The listing builds one solid part. Answer for the finished solid, in the listing's coordinates (mm). A direction names the side the tool comes from. Coordinates: 2 decimals unless noted, no trailing zeros. Write each loop counter-clockwise with the first axis right and the second up, starting at its lowest first coordinate (ties: lowest second). Pieces come first, ordered by that corner, then holes.
```python
from build123d import *

# Parameters (mm, degrees)
F1_DEPTH  = 5
F3_DEPTH  = 5.5
F5_DEPTH  = 5.5
F6_R      = 22.5
F7_DEPTH  = 10.5
F8_R      = 17.5
F9_DEPTH  = 25
F11_DEPTH = 25
F12_R     = 1.25
F13_DEPTH = 11
F14_R     = 2.25
F15_DEPTH = 2.5


with BuildPart() as f1:
    # F0 (on Top) → F1 (new body)
    with BuildSketch(Plane.XY):
        with BuildLine():
            Line((50.7170443075, -14.5414772037), (55.9852813742, -14.5414772037))
            Line((55.9852813742, -14.5414772037), (16.9705627485, 103))
            ThreePointArc((16.9705627485, 103), (8.4852813742, 109), (0, 103))
            Line((0, 103), (-39.0147186258, -14.5414772037))
            Line((-39.0147186258, -14.5414772037), (-33.746481559, -14.5414772037))
            Line((-33.746481559, -14.5414772037), (4.7271265323, 101.3697708508))
            ThreePointArc((4.7271265323, 101.3697708508), (8.4852813742, 104), (12.2434362162, 101.3697708508))
            Line((12.2434362162, 101.3697708508), (50.7170443075, -14.5414772037))
        make_face()
        with BuildLine():
            Line((16.9705627485, 103), (55.9852813742, -14.5414772037))
            Line((55.9852813742, -14.5414772037), (61.253518441, -14.5414772037))
            Line((61.253518441, -14.5414772037), (21.7024158273, 104.6159892602))
            ThreePointArc((21.7024158273, 104.6159892602), (8.4852813742, 114), (-4.7318530788, 104.6159892602))
            Line((-4.7318530788, 104.6159892602), (-44.2829556925, -14.5414772037))
            Line((-44.2829556925, -14.5414772037), (-39.0147186258, -14.5414772037))
            Line((-39.0147186258, -14.5414772037), (0, 103))
            ThreePointArc((0, 103), (8.4852813742, 109), (16.9705627485, 103))
        make_face()
        with BuildLine():
            Line((-33.746481559, -14.5414772037), (50.7170443075, -14.5414772037))
            Line((50.7170443075, -14.5414772037), (12.2434362162, 101.3697708508))
            ThreePointArc((12.2434362162, 101.3697708508), (8.4852813742, 104), (4.7271265323, 101.3697708508))
            Line((4.7271265323, 101.3697708508), (-33.746481559, -14.5414772037))
        make_face()
    extrude(amount=F1_DEPTH)

    # F2 (on face) → F3 (join)
    with BuildSketch(Plane.XY.offset(5)):
        with BuildLine():
            Line((-39.0147186258, -14.5414772037), (0, 103))
            ThreePointArc((0, 103), (8.4852813742, 109), (16.9705627485, 103))
            Line((16.9705627485, 103), (55.9852813742, -14.5414772037))
            Line((55.9852813742, -14.5414772037), (61.253518441, -14.5414772037))
            Line((61.253518441, -14.5414772037), (21.7024158273, 104.6159892602))
            ThreePointArc((21.7024158273, 104.6159892602), (8.4852813742, 114), (-4.7318530788, 104.6159892602))
            Line((-4.7318530788, 104.6159892602), (-44.2829556925, -14.5414772037))
            Line((-44.2829556925, -14.5414772037), (-39.0147186258, -14.5414772037))
        make_face()
    extrude(amount=F3_DEPTH)

    # F4 (on face) → F5 (join)
    with BuildSketch(Plane.XY.offset(5)):
        with BuildLine():
            ThreePointArc((11.29925422, 101.0399792418), (8.4852813742, 103), (5.6713085285, 101.0399792418))
            Line((5.6713085285, 101.0399792418), (-32.6928341457, -14.5414772037))
            Line((-32.6928341457, -14.5414772037), (-27.424597079, -14.5414772037))
            Line((-27.424597079, -14.5414772037), (8.4852813742, 93.6459020283))
            Line((8.4852813742, 93.6459020283), (44.3951598274, -14.5414772037))
            Line((44.3951598274, -14.5414772037), (49.6633968942, -14.5414772037))
            Line((49.6633968942, -14.5414772037), (11.29925422, 101.0399792418))
        make_face()
    extrude(amount=F5_DEPTH)

    # F6 (on face) → F7 (join)
    with BuildSketch(Plane.XY.offset(5)):
        with BuildLine():
            Line((36.3787330735, 9.6099885954), (27.3452487141, 36.8255916626))
            ThreePointArc((27.3452487141, 36.8255916626), (8.4852813742, 43.9585227963), (-10.3746859657, 36.8255916626))
            Line((-10.3746859657, 36.8255916626), (-19.4081703251, 9.6099885954))
            ThreePointArc((-19.4081703251, 9.6099885954), (8.4852813742, -13.0414772037), (36.3787330735, 9.6099885954))
        make_face()
        with Locations((8.4852813742, 15.4585227963)):
            Circle(F6_R, mode=Mode.SUBTRACT)
    extrude(amount=F7_DEPTH)

    # F8 (on face) → F9 (cut)
    with BuildSketch(Plane.XY.offset(5)):
        with Locations((8.4852813742, 15.4585227963)):
            Circle(F8_R)
    extrude(amount=-F9_DEPTH, mode=Mode.SUBTRACT)

    # F10 (on face) → F11 (cut)
    with BuildSketch(Plane.XY.offset(5)):
        with BuildLine():
            Line((8.4852813742, 77.7740365146), (-1.5945371695, 47.4060932537))
            ThreePointArc((-1.5945371695, 47.4060932537), (8.4852813742, 48.9585227963), (18.5650999179, 47.4060932537))
            Line((18.5650999179, 47.4060932537), (8.4852813742, 77.7740365146))
        make_face()
    extrude(amount=-F11_DEPTH, mode=Mode.SUBTRACT)

    # F12 (on face) → F13 (cut)
    with BuildSketch(Plane.XY.offset(10.5)):
        with Locations((8.4959140697, 97.6459020283)):
            Circle(F12_R)
        with Locations((-1.5147186258, 103.6459020283)):
            Circle(F12_R)
        with Locations((18.4852813742, 103.6459020283)):
            Circle(F12_R)
        with Locations((-10.2829556925, 45.4585227963)):
            Circle(F12_R)
        with Locations((27.253518441, 45.4585227963)):
            Circle(F12_R)
        with Locations((56.753518441, -10.5414772037)):
            Circle(F12_R)
        with Locations((43.753518441, -4.5414772037)):
            Circle(F12_R)
        with Locations((-26.7829556925, -4.5414772037)):
            Circle(F12_R)
        with Locations((-39.7829556925, -10.5414772037)):
            Circle(F12_R)
    extrude(amount=-F13_DEPTH, mode=Mode.SUBTRACT)

    # F14 (on face) → F15 (cut)
    with BuildSketch(Plane(origin=(0, 0, 0), x_dir=(1, 0, 0), z_dir=(0, 0, -1))):
        with Locations((18.4852813742, -103.6459020283)):
            Circle(F14_R)
        with Locations((8.4959140697, -97.6459020283)):
            Circle(F14_R)
        with Locations((-1.5147186258, -103.6459020283)):
            Circle(F14_R)
        with Locations((-10.2829556925, -45.4585227963)):
            Circle(F14_R)
        with Locations((27.253518441, -45.4585227963)):
            Circle(F14_R)
        with Locations((-39.7829556925, 10.5414772037)):
            Circle(F14_R)
        with Locations((-26.7829556925, 4.5414772037)):
            Circle(F14_R)
        with Locations((43.753518441, 4.5414772037)):
            Circle(F14_R)
        with Locations((56.753518441, 10.5414772037)):
            Circle(F14_R)
    extrude(amount=-F15_DEPTH, mode=Mode.SUBTRACT)


solid = f1.part
```
(1) Find the intervals of material crossed by probe 1 along X at (y, z) = (71.5, 7); probe 2 along X at (y, z) = (29.5, 9.25); probe 3 along Z at (x, y) = (18, 61.5), in increasing order.
(2) Section A-A, the plane z = 8 is taken. State how many separate pieces and enclosed holes the cut face has, plus the area to 3 significant figures.
(3) Section C-C, the plane y = 58 is taken. Write down the section's boundary in (x, z).
(4) Section B-B, the plane y = 17.5 is taken. Write down the section's boundary in (x, z), plus the area to 3 significant figures.
(5) Which of the six approach directions +Z, -Z, +X, -X, +Y, -Y give full straight-line access (tool end or side, diameter ignored) to faces 4 (the flat face through (29, 45, 2.5)), 5 (the flat face through (40.33, -2.3, 7.71)), 6 (the cylindrical face through (8.3, 109, 7.7))?
(6) Each of these flat-tipped pins is pushed along its axis until it touches: pin 1 (3 mm diameter, centred on x = 56.75, y = -10.54, fed in from -Z); pin 2 (1.5 mm diameter, centred on x = 5, z = 14, fed in from -Y); pin 3 (2 mm diameter, centred on x = 43.75, y = -4.54, fed in from +Z); pin 4 (2 mm diameter, centred on x = 15.5, y = 31, fed in from +Z). Where does it stop, or does it pass through?
(7) For a pull along X with two mould halves and no side action, classify faces 1 (the flat face through (13.596, 62.377, 2.535)), 2 (the flat face through (-4, -14.541, 3)), 3 (the flat face through (-14.828, 23.408, 12.965)) as pulls with the +X half, pulls with the -X half, needs draft (parallel to the pull), parting line crosses it, or undercut.
Solution:
1. probe 1: x = -15.72 to -10.46, -4.13 to 1.13, 15.84 to 21.1, 27.43 to 32.69
1. probe 2: x = -29.66 to -24.4, -18.07 to -9.1, 26.07 to 35.05, 41.37 to 46.64
1. probe 3: z = 0 to 5
2. separate pieces: 2
2. enclosed holes: 11
2. area: 3,360 mm2
3. outline: (-20.2, 0) - (1.92, 0) - (1.92, 5) - (-3.35, 5) - (-3.35, 10.5) - (-8.61, 10.5) - (-8.61, 5) - (-14.94, 5) - (-14.94, 10.5) - (-20.2, 10.5) - close; (15.05, 0) - (37.18, 0) - (37.18, 10.5) - (31.91, 10.5) - (31.91, 5) - (25.59, 5) - (25.59, 10.5) - (20.32, 10.5) - (20.32, 5) - (15.05, 5) - close
4. outline: (-33.65, 0) - (-8.9, 0) - (-8.9, 5) - (-13.92, 5) - (-13.92, 15.5) - (-16.79, 15.5) - (-16.79, 10.5) - (-22.06, 10.5) - (-22.06, 5) - (-28.38, 5) - (-28.38, 10.5) - (-33.65, 10.5) - close; (25.87, 0) - (50.62, 0) - (50.62, 10.5) - (45.35, 10.5) - (45.35, 5) - (39.03, 5) - (39.03, 10.5) - (33.76, 10.5) - (33.76, 15.5) - (30.89, 15.5) - (30.89, 5) - (25.87, 5) - close
4. area: 424 mm2
5. face 4: -Z
5. face 5: +Z, -Y
5. face 6: +Z
6. pin 1: stops at z = 2.5
6. pin 2: stops at y = -12.91
6. pin 3: passes through
6. pin 4: stops at z = 5
7. face 1: undercut
7. face 2: needs draft
7. face 3: pulls with the -X half
